Read the model definition and answer for the solid it produces. Units are mm, in the model's axes. Give positions to 0.01 mm unless a question says otherwise; leave off trailing zeros. Write each loop counter-clockwise with the first axis right and the second up, starting at its lowest first coordinate (ties: lowest second). Pieces come first, ordered by that corner, then holes. Notation, with made-up numbers: (52.25, -29.75) -> (103.25, -29.75) arc R13 ccw to (103.25, -12.75) -> close; hole circle Ø7 at (60, 0.5). An arc over 180 degrees is marked (long way). Write item = value, one per line.
from build123d import *

# Parameters (mm, degrees)
EXTRUDE_1_DEPTH          = 0.5
EXTRUDE_2_DEPTH          = 104.5
SKETCH_8_W               = 60
SKETCH_8_H               = 8
SKETCH_8_W_2             = 60.005961803
CUT_EXTRUDE_2_DEPTH      = 10
CUT_EXTRUDE_3_DEPTH      = 10
EXTRUDE_4_DEPTH          = 2.5
FILLET_3_R               = 0.25
FILLET_4_R               = 0.25
SKETCH_7_R               = 3.5
SKETCH_7_R_2             = 0.5
CUT_EXTRUDE_4_DEPTH      = 244
SKETCH_11_W              = 182.233952392
SKETCH_11_H              = 62.441724199
CUT_EXTRUDE_5_DEPTH      = 3
SKETCH_12_W              = 153.34351729
SKETCH_12_H              = 66.332199781
CUT_EXTRUDE_6_DEPTH      = 3
CUT_EXTRUDE_7_DEPTH      = 164
CUT_EXTRUDE_7_DEPTH_BACK = 90
SKETCH_13_W              = 225.919069127
SKETCH_13_H              = 66.171542843
SKETCH_14_W              = 3
SKETCH_14_H              = 15
EXTRUDE_5_DEPTH          = 1
SKETCH_18_W              = 3
SKETCH_18_H              = 204
EXTRUDE_6_DEPTH          = 4
SKETCH_19_W              = 3
SKETCH_19_H              = 15
SKETCH_19_H_2            = 10
EXTRUDE_7_DEPTH          = 3


with BuildPart() as part:
    # Sketch 1 → Extrude 1 (new body)
    with BuildSketch(Plane.XY):
        Polygon((0, -1.078212291), (0, -59.078212291), (150, -59.078212291), (150, -56.078212291), (24.720670391, -21.433997855), (24.720670391, -1.078212291), align=None)
    extrude(amount=EXTRUDE_1_DEPTH)

    # Sketch 2 → Extrude 2 (add)
    with BuildSketch(Plane(origin=(0, 0, 0), x_dir=(-1, 0, 0), z_dir=(0, 0, -1))):
        with BuildLine():
            Line((0, -1.078212291), (-3, -1.078212291))
            Line((-3, -1.078212291), (-3, -54.078212291))
            Line((-3, -54.078212291), (-149.757649478, -58.570793397))
            ThreePointArc((-149.757649478, -58.570793397), (-149.929460817, -58.646625155), (-150, -58.820676341))
            Line((-150, -58.820676341), (-150, -58.828212291))
            ThreePointArc((-150, -58.828212291), (-149.926776695, -59.004988986), (-149.75, -59.078212291))
            Line((-149.75, -59.078212291), (0, -59.078212291))
            Line((0, -59.078212291), (0, -1.078212291))
        make_face()
    extrude(amount=EXTRUDE_2_DEPTH)

    # Mirror 3: part across plane


with BuildPart() as part_1:
    add(part.part)
    add(part.part.mirror(Plane(origin=(149.75, -58.820676341, -104.5), x_dir=(1, 0, 0), z_dir=(0, 0, 1))))

    # Sketch 8 → Cut-Extrude 2 (cut)
    with BuildSketch(Plane(origin=(-1.651096891, -53.935831773, 0), x_dir=(0.9995317742895511, -0.03059791145784333, 0), z_dir=(0.03059791145784333, 0.9995317742895511, 0))):
        with Locations((121.479673046, 5)):
            Rectangle(SKETCH_8_W, SKETCH_8_H)
        with Locations((121.476692145, 15)):
            Rectangle(SKETCH_8_W_2, SKETCH_8_H)
        with Locations((121.476692145, 24.421052632)):
            Rectangle(SKETCH_8_W_2, SKETCH_8_H)
        with Locations((121.476692145, 33.842105263)):
            Rectangle(SKETCH_8_W_2, SKETCH_8_H)
        with Locations((121.476692145, 43.263157895)):
            Rectangle(SKETCH_8_W_2, SKETCH_8_H)
        with Locations((121.476692145, 52.684210526)):
            Rectangle(SKETCH_8_W_2, SKETCH_8_H)
        with Locations((121.476692145, 62.105263158)):
            Rectangle(SKETCH_8_W_2, SKETCH_8_H)
        with Locations((121.476692145, 71.526315789)):
            Rectangle(SKETCH_8_W_2, SKETCH_8_H)
        with Locations((121.476692145, 80.947368421)):
            Rectangle(SKETCH_8_W_2, SKETCH_8_H)
        with Locations((121.476692145, 90.368421053)):
            Rectangle(SKETCH_8_W_2, SKETCH_8_H)
        with Locations((121.476692145, 99.789473684)):
            Rectangle(SKETCH_8_W_2, SKETCH_8_H)
        with Locations((121.476692145, 109.210526316)):
            Rectangle(SKETCH_8_W_2, SKETCH_8_H)
        with Locations((121.476692145, 118.631578947)):
            Rectangle(SKETCH_8_W_2, SKETCH_8_H)
        with Locations((121.476692145, 128.052631579)):
            Rectangle(SKETCH_8_W_2, SKETCH_8_H)
        with Locations((121.476692145, 137.473684211)):
            Rectangle(SKETCH_8_W_2, SKETCH_8_H)
        with Locations((121.476692145, 146.894736842)):
            Rectangle(SKETCH_8_W_2, SKETCH_8_H)
        with Locations((121.476692145, 156.315789474)):
            Rectangle(SKETCH_8_W_2, SKETCH_8_H)
        with Locations((121.476692145, 165.736842105)):
            Rectangle(SKETCH_8_W_2, SKETCH_8_H)
        with Locations((121.476692145, 175.157894737)):
            Rectangle(SKETCH_8_W_2, SKETCH_8_H)
        with Locations((121.476692145, 184.578947368)):
            Rectangle(SKETCH_8_W_2, SKETCH_8_H)
        with Locations((121.476692145, 194)):
            Rectangle(SKETCH_8_W_2, SKETCH_8_H)
        with Locations((121.479673046, 204)):
            Rectangle(SKETCH_8_W, SKETCH_8_H)
    extrude(amount=-CUT_EXTRUDE_2_DEPTH, mode=Mode.SUBTRACT)

    # Sketch 9 → Cut-Extrude 3 (cut)
    with BuildSketch(Plane(origin=(-1.651096891, -53.935831773, 0), x_dir=(0.9995317742895511, -0.03059791145784333, 0), z_dir=(0.03059791145784333, 0.9995317742895511, 0))):
        Polygon((151.645642318, 209), (153.085665737, 209), (154.855962757, 1), (151.716207414, 1), (151.479673046, 1), (151.479673046, 209), align=None)
    extrude(amount=-CUT_EXTRUDE_3_DEPTH, mode=Mode.SUBTRACT)

    # Sketch 1_3 → Extrude 4 (add)
    with BuildSketch(Plane.XY):
        Polygon((0, -1.078212291), (0, -59.078212291), (150, -59.078212291), (150, -56.078212291), (24.720670391, -21.433997855), (24.720670391, -1.078212291), align=None)
    extrude_4 = extrude(amount=-EXTRUDE_4_DEPTH)

    # Fillet 3
    fillet_3_edges = [part_1.edges().sort_by_distance(p)[0] for p in [
        (149.757649478, -58.570793397, -208.5),
        (149.757649478, -58.570793397, -199),
        (149.757649478, -58.570793397, -189.289473684),
        (149.757649478, -58.570793397, -179.868421053),
        (149.757649478, -58.570793397, -170.447368421),
        (149.757649478, -58.570793397, -161.026315789),
        (149.757649478, -58.570793397, -151.605263158),
        (149.757649478, -58.570793397, -142.184210526),
        (149.757649478, -58.570793397, -132.763157895),
        (149.757649478, -58.570793397, -123.342105263),
        (149.757649478, -58.570793397, -113.921052632),
        (149.757649478, -58.570793397, -104.5),
        (149.757649478, -58.570793397, -95.078947368),
        (149.757649478, -58.570793397, -85.657894737),
        (149.757649478, -58.570793397, -76.236842105),
        (149.757649478, -58.570793397, -66.815789474),
        (149.757649478, -58.570793397, -57.394736842),
        (149.757649478, -58.570793397, -47.973684211),
        (149.757649478, -58.570793397, -38.552631579),
        (149.757649478, -58.570793397, -29.131578947),
        (149.757649478, -58.570793397, -19.710526316),
        (149.757649478, -58.570793397, -10),
    ]]
    fillet(fillet_3_edges, radius=FILLET_3_R)

    # Fillet 4
    fillet_4_edges = [part_1.edges().sort_by_distance(p)[0] for p in [
        (149.742116246, -59.078212291, -208.5),
        (149.742116246, -59.078212291, -199),
        (149.742116246, -59.078212291, -189.289473684),
        (149.742116246, -59.078212291, -179.868421053),
        (149.742116246, -59.078212291, -170.447368421),
        (149.742116246, -59.078212291, -161.026315789),
        (149.742116246, -59.078212291, -151.605263158),
        (149.742116246, -59.078212291, -142.184210526),
        (149.742116246, -59.078212291, -132.763157895),
        (149.742116246, -59.078212291, -123.342105263),
        (149.742116246, -59.078212291, -113.921052632),
        (149.742116246, -59.078212291, -104.5),
        (149.742116246, -59.078212291, -95.078947368),
        (149.742116246, -59.078212291, -85.657894737),
        (149.742116246, -59.078212291, -76.236842105),
        (149.742116246, -59.078212291, -66.815789474),
        (149.742116246, -59.078212291, -57.394736842),
        (149.742116246, -59.078212291, -47.973684211),
        (149.742116246, -59.078212291, -38.552631579),
        (149.742116246, -59.078212291, -29.131578947),
        (149.742116246, -59.078212291, -19.710526316),
        (149.742116246, -59.078212291, -10),
    ]]
    fillet(fillet_4_edges, radius=FILLET_4_R)

    # Mirror 4: Extrude 4 across plane
    add(extrude_4.mirror(Plane(origin=(0, 0, -104.5), x_dir=(1, 0, 0), z_dir=(0, 0, -1))))

    # Sketch 7 → Cut-Extrude 4 (cut)
    with BuildSketch(Plane.XY.offset(0.5)):
        with Locations(Location((8, -45.078212291, 0), (0, 0, 180))):
            Circle(SKETCH_7_R)
        with Locations(Location((25, -45.078212291, 0), (0, 0, 180))):
            Circle(SKETCH_7_R_2)
        with Locations(Location((23, -45.078212291, 0), (0, 0, 180))):
            Circle(SKETCH_7_R_2)
    extrude(amount=-CUT_EXTRUDE_4_DEPTH, mode=Mode.SUBTRACT)

    # Sketch 11 → Cut-Extrude 5 (cut)
    with BuildSketch(Plane.XY.offset(0.5)):
        with Locations((91.116976196, -27.857350192)):
            Rectangle(SKETCH_11_W, SKETCH_11_H)
    extrude(amount=-CUT_EXTRUDE_5_DEPTH, mode=Mode.SUBTRACT)

    # Sketch 12 → Cut-Extrude 6 (cut)
    with BuildSketch(Plane(origin=(0, 0, -209.5), x_dir=(-1, 0, 0), z_dir=(0, 0, -1))):
        with Locations((-76.671758645, -25.912112401)):
            Rectangle(SKETCH_12_W, SKETCH_12_H)
    extrude(amount=-CUT_EXTRUDE_6_DEPTH, mode=Mode.SUBTRACT)

    # Sketch 13 → Cut-Extrude 7 (cut, two sides: drawn at the far end of the back side and taken through both)
    with BuildSketch(Plane(origin=(3, 0, 0), x_dir=(0, 0, -1), z_dir=(1, 0, 0)).offset(-CUT_EXTRUDE_7_DEPTH_BACK)):
        with Locations((115.459534564, -87.163983712)):
            Rectangle(SKETCH_13_W, SKETCH_13_H)
    extrude(amount=CUT_EXTRUDE_7_DEPTH + CUT_EXTRUDE_7_DEPTH_BACK, mode=Mode.SUBTRACT)

    # Sketch 14 → Extrude 5 (add)
    with BuildSketch(Plane.XZ.offset(54.078212291)):
        with Locations((1.5, -40)):
            Rectangle(SKETCH_14_W, SKETCH_14_H)
        with Locations((1.5, -169)):
            Rectangle(SKETCH_14_W, SKETCH_14_H)
    extrude(amount=EXTRUDE_5_DEPTH)

    # Sketch 18 → Extrude 6 (add)
    with BuildSketch(Plane(origin=(0, -1.078212291, 0), x_dir=(1, 0, 0), z_dir=(0, 1, 0))):
        with Locations((1.5, 104.5)):
            Rectangle(SKETCH_18_W, SKETCH_18_H)
    extrude(amount=EXTRUDE_6_DEPTH)

    # Sketch 19 → Extrude 7 (add)
    with BuildSketch(Plane.XY.offset(-2.5)):
        with Locations((1.5, -4.578212291)):
            Rectangle(SKETCH_19_W, SKETCH_19_H)
        with Locations((1.5, -27.078212291)):
            Rectangle(SKETCH_19_W, SKETCH_19_H_2)
    extrude_7 = extrude(amount=EXTRUDE_7_DEPTH)

    # Mirror 5: Extrude 7 across plane
    add(extrude_7.mirror(Plane(origin=(0, 0, -104.5), x_dir=(1, 0, 0), z_dir=(0, 0, -1))))


solid = part_1.part
(1) Given P1, Ø0.9, axis at x = 1.5, z = -207.5, coming from the -Y side; P2, Ø1.5, axis at x = 2, z = -21.5, coming from the -Y side; P3, Ø0.8, axis at x = 1.5, y = -55, coming from the +Z side, each flat-ended and moving along its own axis, determine where each tip first touches the part or whether it passes through.
Checks:
P1 = -32.08
P2 = -54.08
P3 = -32.5
(2) The part is cut by section A-A on x = 2.25. Determine the outline of the cut face in (y, z), plus the area to 3 significant figures.
Checks:
outline = (-55.08, -176.5) -> (-54.08, -176.5) -> (-54.08, -206.5) -> (-32.08, -206.5) -> (-32.08, -209.5) -> (-22.08, -209.5) -> (-22.08, -206.5) -> (-12.08, -206.5) -> (-12.08, -209.5) -> (2.92, -209.5) -> (2.92, 0.5) -> (-12.08, 0.5) -> (-12.08, -2.5) -> (-22.08, -2.5) -> (-22.08, 0.5) -> (-32.08, 0.5) -> (-32.08, -2.5) -> (-54.08, -2.5) -> (-54.08, -32.5) -> (-55.08, -32.5) -> (-55.08, -47.5) -> (-54.08, -47.5) -> (-54.08, -161.5) -> (-55.08, -161.5) -> close
area = 11,800 mm²
(3) Consider L1, parallel to Y at x = 0.85, z = -113; L2, parallel to Z at x = 0.95, y = -33.5. Determine where each line is inside the solid, lowest interval first.
Checks:
L1 = -54.08 to 2.92
L2 = -206.5 to -2.5
(4) The part is cut by section B-B on y = -42. Determine the outline of the cut face in (x, z).
Checks:
outline = (0, -206.5) -> (3, -206.5) -> (3, -2.5) -> (0, -2.5) -> close
(5) The part is cut by section C-C on z = -24. Determine the outline of the cut face in (x, y).
Checks:
outline = (0, -54.08) -> (3, -54.08) -> (3, 2.92) -> (0, 2.92) -> close
